Can you work these out from the model? Positions are in its coordinate system, mm. A direction names the side the tool comes from. Give positions to 0.01 mm unless a question says otherwise; leave off trailing zeros. Loops run counter-clockwise (first coordinate to the right, second up) from the corner with the lowest first, then second, coordinate; pieces in that order, holes last. Notation, with made-up numbers: (82, -9) - (118, -9) arc R31 ccw to (118, 23) - close; hole circle Ø1 at (3, 27.5). An arc over 180 degrees is marked (long way). Answer as a JSON object with one key per item and string values.
```python
from build123d import *

# Parameters (mm, degrees)
F0_W     = 600
F0_H     = 500
F1_DEPTH = 225
F2_T     = -2
F3_W     = 600
F3_H     = 500
F3_W_2   = 568
F3_H_2   = 470
F4_DEPTH = 2
F6_D     = 7
F8_D     = 7
F8_DEPTH = 18
F9_R     = 2


with BuildPart() as f1:
    # F0 (on Front) → F1 (new body)
    with BuildSketch(Plane.XZ):
        with Locations((0, -50)):
            Rectangle(F0_W, F0_H)
    extrude(amount=-F1_DEPTH)

    # F2
    f2_openings = [f1.faces().sort_by_distance(p)[0] for p in [
        (0, 0, -50),
    ]]
    offset(amount=F2_T, openings=f2_openings)

    # F3 (on Front) → F4 (join)
    with BuildSketch(Plane.XZ):
        with Locations((0, -50)):
            Rectangle(F3_W, F3_H)
        with Locations((1, -50)):
            Rectangle(F3_W_2, F3_H_2, mode=Mode.SUBTRACT)
    extrude(amount=F4_DEPTH)

    # F6 (through all)
    with Locations(Plane.XZ.offset(-223)):
        with Locations((-200, 125), (200, 125), (235, -50), (-235, -50)):
            Hole(F6_D / 2)

    # F8
    with Locations(Plane(origin=(0, 0, -300), x_dir=(1, 0, 0), z_dir=(0, 0, -1))):
        with Locations((150, -30), (-150, -30)):
            Hole(F8_D / 2, depth=F8_DEPTH)

    # F9
    f9_edges = [f1.edges().sort_by_distance(p)[0] for p in [
        (0, -2, 200),
        (300, 111.5, 200),
        (0, 225, 200),
        (-300, 111.5, 200),
        (0, -2, -300),
        (0, 225, -300),
        (-300, 111.5, -300),
        (300, 111.5, -300),
        (300, 225, -50),
        (300, -2, -50),
        (-300, 225, -50),
    ]]
    fillet(f9_edges, radius=F9_R)


solid = f1.part
```
1) Imagine slicing it at B-B on z = 60. Write out the boundary of the cut face in (x, y).
Check sheet entries:
{"outline": "(-300, -2) - (-283, -2) - (-283, 0) - (-298, 0) - (-298, 223) - (298, 223) - (298, 0) - (285, 0) - (285, -2) - (298, -2) arc R2 ccw to (300, 0) - (300, 223) arc R2 ccw to (298, 225) - (-298, 225) arc R2 ccw to (-300, 223) - close"}
2) I need wall thicknesses on L1, parallel to Z at x = -5, y = 150.5; L2, parallel to X at y = 154, z = 57; L3, parallel to Y at x = -4.5, z = -236.5. Which ranges of each line are inside material? Lowest first, please.
Check sheet entries:
{"L1": "-300 to -298, 198 to 200", "L2": "-300 to -298, 298 to 300", "L3": "223 to 225"}
3) Imagine slicing it at A-A on y = 205. Write out the boundary of the cut face in (x, z), and give its area (3 significant figures).
Check sheet entries:
{"outline": "(-300, -298) arc R2 ccw to (-298, -300) - (298, -300) arc R2 ccw to (300, -298) - (300, 198) arc R2 ccw to (298, 200) - (-298, 200) arc R2 ccw to (-300, 198) - close; hole (-298, -298) - (298, -298) - (298, 198) - (-298, 198) - close", "area": "4,380 mm2"}
4) If we mould it in two halves opening along Z, with no side actions, what happens to faces 1 (the flat face through (-4, 113, 200)), 2 (the flat face through (-4, 225, -47)), 3 (the flat face through (298, 110, -53)), 4 (the flat face through (-4, 113, -300))? For each: released by +Z, released by -Z, zero draft, split by the parting line, or undercut.
Check sheet entries:
{"face 1": "released by +Z", "face 2": "zero draft", "face 3": "undercut", "face 4": "released by -Z"}
5) Which directions (+Z, -Z, +X, -X, +Y, -Y) give clear straight access to the entire face, cutting with the end or side of a thin tool? Please do faces 5 (the flat face through (-300, 112, -53)), 6 (the flat face through (-4, 110, -298)).
Check sheet entries:
{"face 5": "+Z, -Z, -X, +Y, -Y", "face 6": "none"}
6) I'm going to push flat-ended pins straight in: P1, Ø1, axis at x = -145, z = -22, coming from the -Y side; P2, Ø1.6, axis at x = 49, y = -1.5, coming from the +Z side; P3, Ø1.6, axis at y = -1.5, z = 0.5, coming from the +X side. Where does each tip first touch, or does it pass through?
Check sheet entries:
{"P1": "y = 223", "P2": "z = 199.87", "P3": "x = 299.87"}
7) Imagine slicing it at C-C on x = 86. Write out the boundary of the cut face in (y, z), and give its area (3 significant figures).
Check sheet entries:
{"outline": "(-2, -298) arc R2 ccw to (0, -300) - (223, -300) arc R2 ccw to (225, -298) - (225, 198) arc R2 ccw to (223, 200) - (0, 200) arc R2 ccw to (-2, 198) - (-2, 185) - (0, 185) - (0, 198) - (223, 198) - (223, -298) - (0, -298) - (0, -285) - (-2, -285) - close", "area": "1,950 mm2"}
